Build history of the part. All positions in model axes, mm. Face numbers are marked on the shaded views. A direction names the side the tool comes from. Coordinates: 2 decimals unless noted, no trailing zeros. Order: outer loops, then holes, each group sorted by start corner. A loop starts at its lowest first (then second) coordinate and runs counter-clockwise, first axis right, second up. Notation, with made-up numbers: (39, 82.25) -> (58, 82.25) arc R19 cw to (58, 113.25) -> close; hole circle Ø1 at (53, 73). An arc over 180 degrees is marked (long way). Write each question's results on one line, items separated by ' | '.
from build123d import *

# Parameters (mm, degrees)
SKETCH1_W             = 52.9
SKETCH1_H             = 30
SKETCH1_R             = 10.25
BOSS_EXTRUDE1_DEPTH   = 5
SKETCH2_W             = 52.9
SKETCH2_H             = 30
SKETCH2_W_2           = 43.9
SKETCH2_H_2           = 21
BOSS_EXTRUDE2_DEPTH   = 11.1
SKETCH3_R             = 8.25
CUT_EXTRUDE1_DEPTH    = 53.9
SKETCH4_W             = 52.9
SKETCH4_H             = 5
BOSS_EXTRUDE3_DEPTH   = 15
SKETCH5_W             = 52.9
SKETCH5_H             = 5
BOSS_EXTRUDE4_DEPTH   = 15
SKETCH7_R             = 14.75
SKETCH7_R_2           = 10.25
BOSS_EXTRUDE5_DEPTH   = 15
SKETCH8_R             = 14.75
SKETCH8_R_2           = 1.65
BOSS_EXTRUDE6_DEPTH   = 5
SKETCH9_R             = 8
SKETCH9_R_2           = 3
BOSS_EXTRUDE7_DEPTH   = 5
SKETCH10_W            = 52.9
SKETCH10_H            = 15
BOSS_EXTRUDE8_DEPTH   = 11.1
SKETCH12_R            = 5
CUT_EXTRUDE2_DEPTH    = 8
SKETCH13_R            = 2.2
CUT_EXTRUDE3_DEPTH    = 9.1
BOSS_EXTRUDE11_DEPTH  = 20
SKETCH16_R            = 2.5
CUT_EXTRUDE4_DEPTH    = 5
M3_TAPPED_HOLE1_D     = 2.5
M3_TAPPED_HOLE1_DEPTH = 10.748924226
M3_TAPPED_HOLE1_TIP   = 0.751075774


with BuildPart() as part:
    # Sketch1 → Boss-Extrude1 (new body)
    with BuildSketch(Plane(origin=(0, 0, 0), x_dir=(1, 0, 0), z_dir=(0, 1, 0))):
        Rectangle(SKETCH1_W, SKETCH1_H)
        Circle(SKETCH1_R, mode=Mode.SUBTRACT)
    extrude(amount=BOSS_EXTRUDE1_DEPTH)

    # Sketch2 → Boss-Extrude2 (add)
    with BuildSketch(Plane.XZ):
        Rectangle(SKETCH2_W, SKETCH2_H)
        Rectangle(SKETCH2_W_2, SKETCH2_H_2, mode=Mode.SUBTRACT)
    extrude(amount=BOSS_EXTRUDE2_DEPTH)

    # Sketch3 → Cut-Extrude1 (cut, through all)
    with BuildSketch(Plane(origin=(26.45, 0, 0), x_dir=(0, 0, -1), z_dir=(1, 0, 0))):
        with Locations((0, -11.1)):
            Circle(SKETCH3_R)
    extrude(amount=-CUT_EXTRUDE1_DEPTH, mode=Mode.SUBTRACT)

    # Sketch4 → Boss-Extrude3 (add)
    with BuildSketch(Plane(origin=(0, 0, -15), x_dir=(-1, 0, 0), z_dir=(0, 0, -1))):
        with Locations((0, -8.6)):
            Rectangle(SKETCH4_W, SKETCH4_H)
    extrude(amount=BOSS_EXTRUDE3_DEPTH)

    # Sketch5 → Boss-Extrude4 (add)
    with BuildSketch(Plane.XY.offset(15)):
        with Locations((0, -8.6)):
            Rectangle(SKETCH5_W, SKETCH5_H)
    extrude(amount=BOSS_EXTRUDE4_DEPTH)

    # Sketch7 → Boss-Extrude5 (add)
    with BuildSketch(Plane(origin=(0, 5, 0), x_dir=(1, 0, 0), z_dir=(0, 1, 0))):
        Circle(SKETCH7_R)
        Circle(SKETCH7_R_2, mode=Mode.SUBTRACT)
    extrude(amount=BOSS_EXTRUDE5_DEPTH)

    # Sketch8 → Boss-Extrude6 (add)
    with BuildSketch(Plane(origin=(0, 20, 0), x_dir=(1, 0, 0), z_dir=(0, 1, 0))):
        Circle(SKETCH8_R)
        Circle(SKETCH8_R_2, mode=Mode.SUBTRACT)
    extrude(amount=BOSS_EXTRUDE6_DEPTH)

    # Sketch9 → Boss-Extrude7 (add)
    with BuildSketch(Plane(origin=(0, 25, 0), x_dir=(1, 0, 0), z_dir=(0, 1, 0))):
        Circle(SKETCH9_R)
        Circle(SKETCH9_R_2, mode=Mode.SUBTRACT)
    extrude(amount=BOSS_EXTRUDE7_DEPTH)

    # Sketch10 → Boss-Extrude8 (add)
    with BuildSketch(Plane(origin=(0, -6.1, 0), x_dir=(1, 0, 0), z_dir=(0, 1, 0))):
        with Locations((0, 22.5)):
            Rectangle(SKETCH10_W, SKETCH10_H)
        with Locations((0, -22.5)):
            Rectangle(SKETCH10_W, SKETCH10_H)
    extrude(amount=BOSS_EXTRUDE8_DEPTH)

    # Sketch12 → Cut-Extrude2 (cut)
    with BuildSketch(Plane(origin=(0, 5, 0), x_dir=(1, 0, 0), z_dir=(0, 1, 0))):
        with Locations((-16.45, -22.5)):
            Circle(SKETCH12_R)
        with Locations((16.45, -22.5)):
            Circle(SKETCH12_R)
        with Locations((16.45, 22.5)):
            Circle(SKETCH12_R)
        with Locations((-16.45, 22.5)):
            Circle(SKETCH12_R)
    extrude(amount=-CUT_EXTRUDE2_DEPTH, mode=Mode.SUBTRACT)

    # Sketch13 → Cut-Extrude3 (cut, through all)
    with BuildSketch(Plane(origin=(0, -3, 0), x_dir=(1, 0, 0), z_dir=(0, 1, 0))):
        with Locations((-16.45, -22.5)):
            Circle(SKETCH13_R)
        with Locations((-16.45, 22.5)):
            Circle(SKETCH13_R)
        with Locations((16.45, 22.5)):
            Circle(SKETCH13_R)
        with Locations((16.45, -22.5)):
            Circle(SKETCH13_R)
    extrude(amount=-CUT_EXTRUDE3_DEPTH, mode=Mode.SUBTRACT)

    # Sketch14 → Boss-Extrude11 (add)
    with BuildSketch(Plane(origin=(0, 5, 0), x_dir=(1, 0, 0), z_dir=(0, 1, 0))):
        with BuildLine():
            Line((-26.45, 14.75), (-26.45, -14.75))
            Line((-26.45, -14.75), (4e-09, -14.75))
            ThreePointArc((4e-09, -14.75), (-14.75, -5e-09), (-6e-09, 14.75))
            Line((-6e-09, 14.75), (-26.45, 14.75))
        make_face()
        with BuildLine():
            ThreePointArc((14.75, 0), (10.429825024, -10.429825021), (4e-09, -14.75))
            Line((4e-09, -14.75), (26.45, -14.75))
            Line((26.45, -14.75), (26.45, 14.75))
            Line((26.45, 14.75), (-6e-09, 14.75))
            ThreePointArc((-6e-09, 14.75), (10.42982502, 10.429825025), (14.75, 0))
        make_face()
    extrude(amount=BOSS_EXTRUDE11_DEPTH)

    # Sketch16 → Cut-Extrude4 (cut)
    with BuildSketch(Plane(origin=(0, 25, 0), x_dir=(1, 0, 0), z_dir=(0, 1, 0))):
        with Locations((18.5, 0)):
            Circle(SKETCH16_R)
        with Locations((-18.5, 0)):
            Circle(SKETCH16_R)
    extrude(amount=-CUT_EXTRUDE4_DEPTH, mode=Mode.SUBTRACT)

    # M3 Tapped Hole1
    with Locations(Plane(origin=(0, 20, 0), x_dir=(1, 0, 0), z_dir=(0, 1, 0))):
        with Locations((-18.5, 0), (18.5, 0)):
            Hole(M3_TAPPED_HOLE1_D / 2, depth=M3_TAPPED_HOLE1_DEPTH)
            with Locations((0, 0, -(M3_TAPPED_HOLE1_DEPTH + M3_TAPPED_HOLE1_TIP / 2))):  # 118° drill point
                Cone(0, M3_TAPPED_HOLE1_D / 2, M3_TAPPED_HOLE1_TIP, mode=Mode.SUBTRACT)


solid = part.part
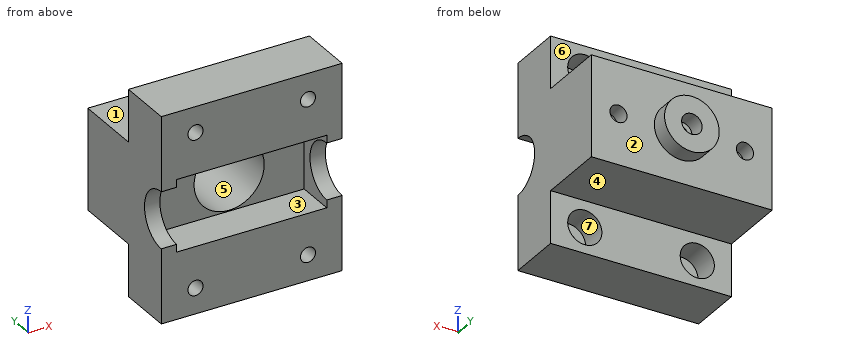
Item 1: Slice it at B-B, the plane x = 0. List the corners of the cut face in (y, z), and give its area (3 significant figures).
Answer:
outline: (-11.1, -30) -> (5, -30) -> (5, -14.75) -> (25, -14.75) -> (25, -8) -> (30, -8) -> (30, -3) -> (25, -3) -> (25, -1.65) -> (20, -1.65) -> (20, -10.25) -> (0, -10.25) -> (0, -10.5) -> (-11.1, -10.5) -> close; (-11.1, 10.5) -> (0, 10.5) -> (0, 10.25) -> (20, 10.25) -> (20, 1.65) -> (25, 1.65) -> (25, 3) -> (30, 3) -> (30, 8) -> (25, 8) -> (25, 14.75) -> (5, 14.75) -> (5, 30) -> (-11.1, 30) -> close | area: 946 mm^2
Item 2: Slice it at C-C, the plane y = 13.5. List the corners of the cut face in (x, z).
Answer:
outline: (-26.45, -14.75) -> (26.45, -14.75) -> (26.45, 14.75) -> (-26.45, 14.75) -> close; hole circle Ø2.5 at (-18.5, 0); hole circle Ø20.5 at (0, 0); hole circle Ø2.5 at (18.5, 0)
Item 3: Tool access for the marked faces 4, 5, 6 and 7: list every direction of +Z, -Z, +X, -X, +Y, -Y with a clear straight run to the whole face (end or side of a thin tool).
Answer:
face 4: -Z, +X, -X, +Y | face 5: -Y | face 6: +Z, +X, -X, +Y | face 7: +Y
Item 4: Slice it at D-D, the plane y = -1.5. List the corners of the cut face in (x, z), and give its area (3 significant figures).
Answer:
outline: (-26.45, -30) -> (26.45, -30) -> (26.45, 30) -> (-26.45, 30) -> close; hole (-21.95, -10.5) -> (21.95, -10.5) -> (21.95, 10.5) -> (-21.95, 10.5) -> close; hole circle Ø10 at (-16.45, -22.5); hole circle Ø10 at (-16.45, 22.5); hole circle Ø10 at (16.45, -22.5); hole circle Ø10 at (16.45, 22.5) | area: 1,940 mm^2
Item 5: Drill centre lines: line 1 (X direction, y = 22.5, z = 0); line 2 (X direction, y = 0, z = 22.5); line 3 (Z direction, x = 16.45, y = -8.25). Where is each one in solid material? Low to high. Write a range as from..to.
Answer:
line 1: x = -26.45..-21, -16..-1.65, 1.65..16, 21..26.45 | line 2: x = -26.45..-21.45, -11.45..11.45, 21.45..26.45 | line 3: z = -30..-24.7, -20.3..-10.5, 10.5..20.3, 24.7..30
Item 6: Slice it at A-A, the plane z = 22.5. List the corners of the cut face in (x, y).
Answer:
outline: (-26.45, -11.1) -> (-18.65, -11.1) -> (-18.65, -3) -> (-21.45, -3) -> (-21.45, 5) -> (-26.45, 5) -> close; (-14.25, -11.1) -> (14.25, -11.1) -> (14.25, -3) -> (11.45, -3) -> (11.45, 5) -> (-11.45, 5) -> (-11.45, -3) -> (-14.25, -3) -> close; (18.65, -11.1) -> (26.45, -11.1) -> (26.45, 5) -> (21.45, 5) -> (21.45, -3) -> (18.65, -3) -> close
Item 7: Pin check, flat tips, straight feed: pin 1 (1.8 mm diameter, centred on x = 0, z = 0.5, fed in from +Y); pin 2 (8 mm diameter, centred on x = -16, z = 23, fed in from +Y); pin 3 (12.5 mm diameter, centred on x = 0, z = 0, fed in from -Y); pin 4 (8 mm diameter, centred on x = -18.5, z = -23, fed in from +Y). Stop position of each tip, or through.
Answer:
pin 1: passes through | pin 2: stops at y = -3 | pin 3: stops at y = 20 | pin 4: stops at y = 5
Item 8: Pull direction Z, two halves, no side cores. Call the marked faces 1, 2 and 3: released by +Z, released by -Z, zero draft, split by the parting line, or undercut.
Answer:
face 1: released by +Z | face 2: zero draft | face 3: undercut
